```python
from build123d import *

# Parameters (mm, degrees)
SKETCH1_W           = 63
SKETCH1_H           = 24
SKETCH1_R           = 3.8
BOSS_EXTRUDE1_DEPTH = 13.53
SKETCH1_3_R         = 2.05
BOSS_EXTRUDE2_DEPTH = 13.53


with BuildPart() as part:
    # Sketch1 → Boss-Extrude1 (new body)
    with BuildSketch(Plane.XY):
        with Locations((0, -2)):
            Rectangle(SKETCH1_W, SKETCH1_H)
        with Locations((-23, 0)):
            Circle(SKETCH1_R, mode=Mode.SUBTRACT)
        with Locations((23, 0)):
            Circle(SKETCH1_R, mode=Mode.SUBTRACT)
    extrude(amount=BOSS_EXTRUDE1_DEPTH)

    # Sketch1_3 → Boss-Extrude2 (add)
    with BuildSketch(Plane.XY):
        Polygon((0, -36.51566868), (13, -36.51566868), (31.5, -14), (-31.5, -14), (-13, -36.51566868), align=None)
        with Locations((0, -31.299955557)):
            Circle(SKETCH1_3_R, mode=Mode.SUBTRACT)
        with Locations((0, -21.322069584)):
            Circle(SKETCH1_3_R, mode=Mode.SUBTRACT)
    extrude(amount=BOSS_EXTRUDE2_DEPTH)


solid = part.part
```
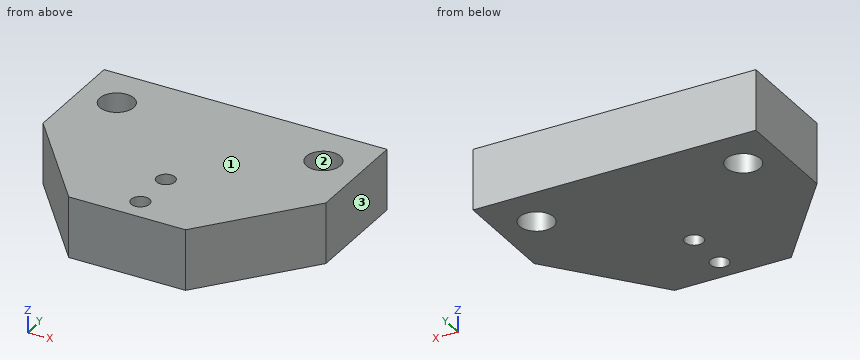
For this review, take the finished solid that the model builds, in its own axes (mm). Face numbers are marked on the shaded views. Coordinates: 2 decimals unless noted, no trailing zeros. Write each loop counter-clockwise with the first axis right and the second up, starting at its lowest first coordinate (ties: lowest second). Pieces come first, ordered by that corner, then holes.
(1) For pin 1 Ø3 at (y, z) = (-30, 1.5) entering from -X; pin 2 Ø7 at (x, y) = (-23, 0) entering from -Z; pin 3 Ø8 at (y, z) = (-24.5, 7) entering from +X, all flat-tipped, find the tip position at first contact; note any pin that passes through.
(2) The part is to be moulded in two halves that separate along X. For the marked faces 1, 2 and 3, say which applies: +X half, -X half, draft (parallel to the pull), parting line (faces both ways), or undercut.
(3) Add section C-C on x = -23. Give the boundary of the cut face in (y, z), then the cut area to 3 significant figures.
(4) Wall thickness on probe 1 along Y at (x, z) = (0, 5); probe 2 along X at (y, z) = (3, 3); probe 3 along X at (y, z) = (-1, 4.75): over which ranges is each line inside the solid? List them lowest first.
(5) Add section D-D on z = 2. Give the boundary of the cut face in (x, y), then the cut area to 3 significant figures.
(6) Add section A-A on y = 0. Give the boundary of the cut face in (x, z).
(7) Add section B-B on x = 0. Give the boundary of the cut face in (y, z), then the cut area to 3 significant figures.
Answer sheet:
1. pin 1: stops at x = -19.59
1. pin 2: passes through
1. pin 3: stops at x = 26.16
2. face 1: draft
2. face 2: undercut
2. face 3: +X half
3. outline: (-24.35, 0) - (-3.8, 0) - (-3.8, 13.53) - (-24.35, 13.53) - close; (3.8, 0) - (10, 0) - (10, 13.53) - (3.8, 13.53) - close
3. area: 362 mm2
4. probe 1: y = -36.52 to -33.35, -29.25 to -23.37, -19.27 to 10
4. probe 2: x = -31.5 to -25.33, -20.67 to 20.67, 25.33 to 31.5
4. probe 3: x = -31.5 to -26.67, -19.33 to 19.33, 26.67 to 31.5
5. outline: (-31.5, -14) - (-13, -36.52) - (13, -36.52) - (31.5, -14) - (31.5, 10) - (-31.5, 10) - close; hole circle Ø7.6 at (-23, 0); hole circle Ø4.1 at (0, -31.3); hole circle Ø4.1 at (0, -21.32); hole circle Ø7.6 at (23, 0)
5. area: 2,400 mm2
6. outline: (-31.5, 0) - (-26.8, 0) - (-26.8, 13.53) - (-31.5, 13.53) - close; (-19.2, 0) - (19.2, 0) - (19.2, 13.53) - (-19.2, 13.53) - close; (26.8, 0) - (31.5, 0) - (31.5, 13.53) - (26.8, 13.53) - close
7. outline: (-36.52, 0) - (-33.35, 0) - (-33.35, 13.53) - (-36.52, 13.53) - close; (-29.25, 0) - (-23.37, 0) - (-23.37, 13.53) - (-29.25, 13.53) - close; (-19.27, 0) - (10, 0) - (10, 13.53) - (-19.27, 13.53) - close
7. area: 518 mm2
